Autodesk Inventor part; units mm, degrees
ref_plane "YZ Plane" through (0, 0, 0) normal (1, 0, 0) x (0, 1, 0)
ref_plane "XZ Plane" through (0, 0, 0) normal (0, 1, 0) x (-1, 0, 0)
ref_plane "XY Plane" through (0, 0, 0) normal (0, 0, 1) x (1, 0, 0)
sketch "Sketch1" plane through (0, 0, 0) normal (0, 0, 1) x (1, 0, 0)
  line L0 (-23.4826, 4.2639) -> (2.3174, 4.2639)
  line L1 (2.3174, 4.2639) -> (2.3174, 2.2639)
  line L2 (2.3174, 2.2639) -> (-23.4826, 2.2639)
  line L3 (-23.4826, 2.2639) -> (-23.4826, 4.2639)
  line L4 (-25.4826, 6.2639) -> (4.3174, 6.2639)
  line L5 (4.3174, 6.2639) -> (4.3174, 0.2639)
  line L6 (4.3174, 0.2639) -> (-25.4826, 0.2639)
  line L7 (-25.4826, 0.2639) -> (-25.4826, 6.2639)
  point P0 (0, 0)
  dimension "d0" = 25.8
  dimension "d1" = 2
  dimension "d4" = 2
  dimension "d5" = 2
  dimension "d6" = 2
  dimension "d7" = 2
extrude "Extrusion5" add sketch "Sketch1" along normal blind 23 contours L0 L1 L2 L3 | L4 L5 L6 L7
sketch "Sketch4" plane through (0, 0, 23) normal (0, 0, 1) x (1, 0, 0)
  line L0 (-23.4826, 4.2639) -> (2.3174, 4.2639)
  line L1 (2.3174, 4.2639) -> (2.3174, 2.2639)
  line L2 (2.3174, 2.2639) -> (-23.4826, 2.2639)
  line L3 (-23.4826, 2.2639) -> (-23.4826, 4.2639)
  line L4 (-25.4826, 6.2639) -> (-25.4826, 0.2639)
  line L5 (4.3174, 6.2639) -> (-25.4826, 6.2639)
  line L6 (-25.4826, 0.2639) -> (4.3174, 0.2639)
  line L7 (4.3174, 0.2639) -> (4.3174, 6.2639)
  point P0 (0, 0)
  dimension "d20" = 2
  dimension "d21" = 2
  dimension "d22" = 2
  dimension "d23" = 2
extrude "Extrusion6" cut sketch "Sketch4" against normal blind 21 contours L0 L1 L2 L3
sketch "Sketch5" plane through (-25.4826, 6.2639, 0) normal (0, 1, 0) x (1, 0, 0)
  line L0 (0, -23) -> (29.8, -23)
  line L1 (4, -4) -> (25.8, -4)
  line L2 (25.8, -4) -> (25.8, -23)
  line L3 (25.8, -23) -> (4, -23)
  line L4 (4, -23) -> (4, -4)
  line L5 (0, 0) -> (0, -23)
  line L6 (29.8, 0) -> (29.8, -23)
  line L7 (0, 0) -> (29.8, 0)
  point P0 (25.4826, 0)
  dimension "d26" = 4
  dimension "d27" = 4
  dimension "d28" = 4
extrude "Extrusion7" cut sketch "Sketch5" against normal through all contours L4 L1 L2 L0
chamfer "Chamfer1" distance 2 angle 45 4 edges at (-21.4826, 5.2639, 4) (-21.4826, 1.2639, 4) (0.3174, 5.2639, 4) (0.3174, 1.2639, 4)
properties part number "CameraHolder"
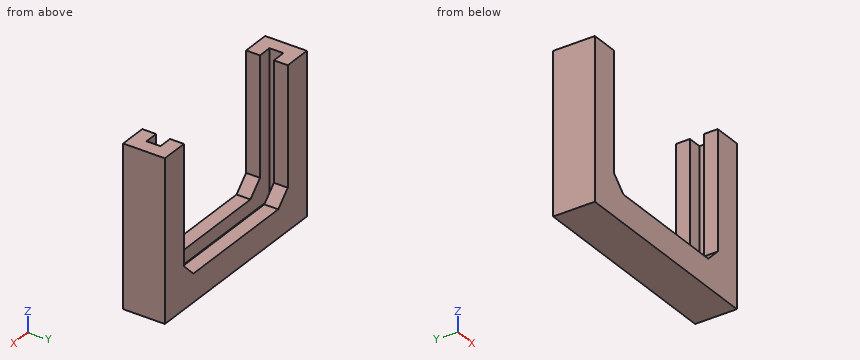
Verification items for the finished model (mm, model axes). Give positions to 0.01 mm unless a question says otherwise; leave off trailing zeros. Order: outer loops, then holes, each group sorted by start corner. A loop starts at its lowest first (then second) coordinate and runs counter-clockwise, first axis right, second up. Notation, with made-up numbers: M 13.5,67.5 L 33.5,67.5 A14 cw 33.5,79.5 Z; hole C 74,24 d2. An arc over 180 degrees is marked long. Answer in a Markdown table with one row per item. Add a question column.
Item 1: Scan lines: probe 1 along X at (y, z) = (3.75, 13.75); probe 2 along X at (y, z) = (5.4, 16.5); probe 3 along Y at (x, z) = (0.75, 15.75). Record each from-to range of solid material in increasing order. Write a range as from..to.
Item 2: Section check A-A, the plane z = 7. Enter the section's corners in (x, y), and give its area (3 significant figures).
Item 3: Section check B-B, the plane x = -5. Enter the section's corners in (y, z), and give its area (3 significant figures).
Item 4: Section check C-C, the plane y = 2.8. Enter the section's corners in (x, z), and give its area (3 significant figures).
Item 5: Gauge pin test, flat end, axial feed: pin 1 (1.6 mm diameter, centred on x = -12, y = 3, fed in from +Z). Record the tip position at first contact, or that the pin passes through.
Item 6: Section check D-D, the plane z = 3.5. Enter the section's corners in (x, y).
Filled sheet:
| question | item | result |
|---|---|---|
| 1 | probe 1 | x = -25.48..-23.48, 2.32..4.32 |
| 1 | probe 2 | x = -25.48..-21.48, 0.32..4.32 |
| 1 | probe 3 | y = 0.26..2.26, 4.26..6.26 |
| 2 | outline | M -25.48,0.26 L -21.48,0.26 L -21.48,2.26 L -23.48,2.26 L -23.48,4.26 L -21.48,4.26 L -21.48,6.26 L -25.48,6.26 Z; M 0.32,0.26 L 4.32,0.26 L 4.32,6.26 L 0.32,6.26 L 0.32,4.26 L 2.32,4.26 L 2.32,2.26 L 0.32,2.26 Z |
| 2 | area | 40.0 mm^2 |
| 3 | outline | M 0.26,0 L 6.26,0 L 6.26,4 L 4.26,4 L 4.26,2 L 2.26,2 L 2.26,4 L 0.26,4 Z |
| 3 | area | 20.0 mm^2 |
| 4 | outline | M -25.48,0 L 4.32,0 L 4.32,23 L 2.32,23 L 2.32,2 L -23.48,2 L -23.48,23 L -25.48,23 Z |
| 4 | area | 144 mm^2 |
| 5 | pin 1 | stops at z = 4 |
| 6 | outline | M -25.48,0.26 L 4.32,0.26 L 4.32,6.26 L -25.48,6.26 Z; hole M -23.48,2.26 L 2.32,2.26 L 2.32,4.26 L -23.48,4.26 Z |
